Geometry: final body of the model. Coordinates: model frame, mm. A direction names the side the tool comes from. Give positions to 0.01 mm unless a question says otherwise; leave off trailing zeros. Order: outer loops, then holes, each group sorted by start corner. A loop starts at its lowest first (then second) coordinate and runs counter-clockwise, first axis right, second up. Notation, with made-up numbers: (25.25, -29.5) -> (53.25, -29.5) arc R11 cw to (53.25, -17.5) -> close; hole circle Ø1 at (59.25, -24.75). An arc over 180 degrees is marked (long way). One line per question, with ' | ' between items. Start each with the question number.
(1) Set-up query: faces 4 (the face through (-0.33, -0.731, -4.493)), 5 (the face through (-1.9, -40.1, 8.9)), 6 (the face through (-7.436, 80.634, 2.024)), 7 (the face through (4, -27, 3)). Return all of +Z, -Z, +X, -X, +Y, -Y with unobstructed straight access to the full face (end or side cutting, diameter ignored); none if empty.
(2) Section B-B (y = -11.5). Return loops of the section in (x, z).
(3) First-contact query: pin 1 Ø2.5 at (y, z) = (83.5, 2.5) entering from +X; pin 2 Ø5 at (x, y) = (8, 62) entering from +Z; pin 3 Ø3 at (y, z) = (55.5, 10.5) entering from +X. Flat tips, straight axial feed; report the tip coordinate or a pass-through.
(4) Section A-A (y = 17.5). Return loops of the section in (x, z), then the cut area to 3 significant figures.
(5) Ray query, L1, parallel to Y at x = 9.75, z = 5; L2, parallel to Y at x = 3, z = 11.25; L3, parallel to X at y = -36, z = 5. Return the intervals inside material, ascending.
(6) Mould query, pull axis Y, two halves, no side actions, for faces 1 (the face through (-0.3, 99.3, -3.6)), 2 (the face through (-0.33, 96.381, -4.493)), 3 (the face through (7.4, 15, 7.5)). Classes: +Y half, -Y half, draft (parallel to the pull), parting line (faces both ways), or undercut.
```python
from build123d import *

# Parameters (mm, degrees)
SFAZOWANIE2_SIZE           = 1
WYTNIJ_WYCI_GNI_CIE1_DEPTH = 5.5
WYTNIJ_WYCI_GNI_CIE2_DEPTH = 6
SFAZOWANIE3_SIZE           = 2


with BuildPart() as part:
    # Szkic1 → Obrót1 (revolve)
    with BuildSketch(Plane(origin=(0, 0, 0), x_dir=(0, 0, -1), z_dir=(1, 0, 0))):
        Polygon((-3, -6.188308688), (-3, 99.409284105), (-10.5, 99.409284105), (-10.5, 94.409284105), (-10.15, 94.409284105), (-10.15, 93.309284105), (-10.5, 93.309284105), (-10.5, 68.309284105), (-15, 68.309284105), (-15, 43.309284105), (-13, 43.309284105), (-13, 36.309284105), (-12.5, 36.309284105), (-12.5, 35.009284105), (-13, 35.009284105), (-13, 28.309284105), (-10.5, 28.309284105), (-10.5, 15), (-13, 15), (-13, 10), (-10.5, 10), (-10.5, 4.778207376), (-9.5, 4.778207376), (-9.5, 3.660040364), (-10.5, 3.660040364), (-10.5, -5), (-9.5, -5), (-9.5, -15.9), (-9.2, -15.9), (-9.2, -17), (-9.5, -17), (-9.5, -39.5), (-9.2, -39.5), (-9.2, -40.6), (-9.5, -40.6), (-9.5, -45), (-3, -45), (-3, -6.690715895), align=None)
    revolve(axis=Axis((0, 99.409284105, 3), (0, -1, 0)))

    # Sfazowanie2
    sfazowanie2_edges = [part.edges().sort_by_distance(p)[0] for p in [
        (0, 10, -7),
        (0, 15, -4.5),
        (0, 28.309284105, -4.5),
        (0, 68.309284105, -9),
        (0, 99.409284105, -4.5),
    ]]
    chamfer(sfazowanie2_edges, length=SFAZOWANIE2_SIZE)

    # Szkic2 → Wytnij-wyciągnięcie1 (cut)
    with BuildSketch(Plane(origin=(10, 0, 0), x_dir=(0, 0, -1), z_dir=(1, 0, 0))):
        with BuildLine():
            Line((-0.5, 87.721044176), (-0.5, 77.721044176))
            ThreePointArc((-0.5, 77.721044176), (-3, 75.221044176), (-5.5, 77.721044176))
            Line((-5.5, 77.721044176), (-5.5, 87.721044176))
            ThreePointArc((-5.5, 87.721044176), (-3, 90.221044176), (-0.5, 87.721044176))
        make_face()
    extrude(amount=-WYTNIJ_WYCI_GNI_CIE1_DEPTH, mode=Mode.SUBTRACT)

    # Szkic2<4> → Wytnij-wyciągnięcie2 (cut)
    with BuildSketch(Plane(origin=(10, 0, 0), x_dir=(0, 0, -1), z_dir=(1, 0, 0))):
        with BuildLine():
            Line((-5.5, -20.047619848), (-5.5, -35.047619848))
            ThreePointArc((-5.5, -35.047619848), (-3, -37.547619848), (-0.5, -35.047619848))
            Line((-0.5, -35.047619848), (-0.5, -20.047619848))
            ThreePointArc((-0.5, -20.047619848), (-3, -17.547619848), (-5.5, -20.047619848))
        make_face()
    extrude(amount=-WYTNIJ_WYCI_GNI_CIE2_DEPTH, mode=Mode.SUBTRACT)

    # Sfazowanie3
    sfazowanie3_edges = [part.edges().sort_by_distance(p)[0] for p in [
        (0, -45, -3.5),
    ]]
    chamfer(sfazowanie3_edges, length=SFAZOWANIE3_SIZE)


solid = part.part
```
Response:
1) face 4: -Y | face 5: none | face 6: +Y | face 7: +X
2) outline: circle Ø13 at (0, 3)
3) pin 1: stops at x = 4.5 | pin 2: stops at z = 13.67 | pin 3: stops at x = 10.39
4) outline: circle Ø15 at (0, 3) | area: 177 mm^2
5) L1: y = 10.95 to 15, 28.31 to 35.01, 36.31 to 68.31 | L2: y = 10 to 15, 28.31 to 68.31 | L3: x = -6.18 to 4
6) face 1: +Y half | face 2: draft | face 3: undercut
